```python
from build123d import *

# Parameters (mm, degrees)
SKETCH_1_R      = 8.5
EXTRUDE_1_DEPTH = 3


with BuildPart() as part:
    # 草图1 → 凸台-拉伸1 (new body)
    with BuildSketch(Plane.XY):
        with BuildLine():
            Line((21.064196615, 7.08036062), (9.146107852, 4.376016947))
            ThreePointArc((9.146107852, 4.376016947), (7.169407686, 7.169407686), (4.376016947, 9.146107852))
            Line((4.376016947, 9.146107852), (7.08036062, 21.064196615))
            Line((7.08036062, 21.064196615), (5.157837228, 21.615471327))
            Line((5.157837228, 21.615471327), (1.135625903, 10.075275031))
            ThreePointArc((1.135625903, 10.075275031), (0, 10.139073584), (-1.135625903, 10.075275031))
            Line((-1.135625903, 10.075275031), (-5.157837228, 21.615471327))
            Line((-5.157837228, 21.615471327), (-7.08036062, 21.064196615))
            Line((-7.08036062, 21.064196615), (-4.376016947, 9.146107852))
            ThreePointArc((-4.376016947, 9.146107852), (-7.169407686, 7.169407686), (-9.146107852, 4.376016947))
            Line((-9.146107852, 4.376016947), (-21.064196615, 7.08036062))
            Line((-21.064196615, 7.08036062), (-21.615471327, 5.157837228))
            Line((-21.615471327, 5.157837228), (-10.075275031, 1.135625903))
            ThreePointArc((-10.075275031, 1.135625903), (-10.139073584, 0), (-10.075275031, -1.135625903))
            Line((-10.075275031, -1.135625903), (-21.615471327, -5.157837228))
            Line((-21.615471327, -5.157837228), (-21.064196615, -7.08036062))
            Line((-21.064196615, -7.08036062), (-9.146107852, -4.376016947))
            ThreePointArc((-9.146107852, -4.376016947), (-7.169407686, -7.169407686), (-4.376016947, -9.146107852))
            Line((-4.376016947, -9.146107852), (-7.08036062, -21.064196615))
            Line((-7.08036062, -21.064196615), (-5.157837228, -21.615471327))
            Line((-5.157837228, -21.615471327), (-1.135625903, -10.075275031))
            ThreePointArc((-1.135625903, -10.075275031), (0, -10.139073584), (1.135625903, -10.075275031))
            Line((1.135625903, -10.075275031), (5.157837228, -21.615471327))
            Line((5.157837228, -21.615471327), (7.08036062, -21.064196615))
            Line((7.08036062, -21.064196615), (4.376016947, -9.146107852))
            ThreePointArc((4.376016947, -9.146107852), (7.169407686, -7.169407686), (9.146107852, -4.376016947))
            Line((9.146107852, -4.376016947), (21.064196615, -7.08036062))
            Line((21.064196615, -7.08036062), (21.615471327, -5.157837228))
            Line((21.615471327, -5.157837228), (10.075275031, -1.135625903))
            ThreePointArc((10.075275031, -1.135625903), (10.139073584, 0), (10.075275031, 1.135625903))
            Line((10.075275031, 1.135625903), (21.615471327, 5.157837228))
            Line((21.615471327, 5.157837228), (21.064196615, 7.08036062))
        make_face()
        Circle(SKETCH_1_R, mode=Mode.SUBTRACT)
    extrude(amount=EXTRUDE_1_DEPTH)


solid = part.part
```
Model file for the job. Use its own axes, mm. A direction names the side the tool comes from. Coordinates: 2 decimals unless noted, no trailing zeros. Order: outer loops, then holes, each group sorted by start corner. A loop starts at its lowest first (then second) coordinate and runs counter-clockwise, first axis right, second up. Notation, with made-up numbers: (61, 77.25) -> (86, 77.25) arc R13 cw to (86, 81.25) -> close; hole circle Ø3 at (40, 14). An arc over 180 degrees is marked (long way). Answer as a JSON object with one key per item and string values. Group by question number.
1) Pull direction Y, two halves, no side cores. Call faces 1 (the face through (-21.344, -6.106, 1.479)), 2 (the face through (-5.71, -15.02, 1.48)), 3 (the face through (0.02, 10.14, 1.48)): +Y half, -Y half, draft (parallel to the pull), parting line (faces both ways), or undercut.
2) Which spindle directions (+Z, -Z, +X, -X, +Y, -Y) get a long thin tool onto all of the face, cutting with end or side? Do faces 4 (the face through (3.119, -15.765, 1.479)), 5 (the face through (-15.02, 5.71, 1.48)), 6 (the face through (-15.765, -3.119, 1.479)), 7 (the face through (-7.2, -7.14, 1.48)). Say none if no direction does.
3) Cut at A-A, the plane x = 0. Write the cut outline in (y, z), then the cut area to 3 significant figures.
4) Drill centre lines: L1, parallel to Y at x = 0, z = 2.05; L2, parallel to Y at x = -18, z = 0.2; L3, parallel to X at y = 17.5, z = 2. Where is each one in solid material? Low to high.
Check values:
{
 "1": {"face 1": "-Y half", "face 2": "undercut", "face 3": "+Y half"},
 "2": {"face 4": "+Z, -Z, -Y", "face 5": "+Z, -Z, +Y", "face 6": "+Z, -Z, -X", "face 7": "+Z, -Z"},
 "3": {"outline": "(-10.14, 0) -> (-8.5, 0) -> (-8.5, 3) -> (-10.14, 3) -> close; (8.5, 0) -> (10.14, 0) -> (10.14, 3) -> (8.5, 3) -> close", "area": "9.83 mm²"},
 "4": {"L1": "y = -10.14 to -8.5, 8.5 to 10.14", "L2": "y = -6.39 to -3.9, 3.9 to 6.39", "L3": "x = -6.27 to -3.72, 3.72 to 6.27"}
}
